Can you work these out from the model? Positions are in its coordinate system, mm. Face numbers are marked on the shaded views. A direction names the side the tool comes from. Round coordinates to 2 decimals unless told otherwise and drop trailing zeros. Loops run counter-clockwise (first coordinate to the right, second up) from the corner with the lowest first, then second, coordinate; pieces in that order, holes last.
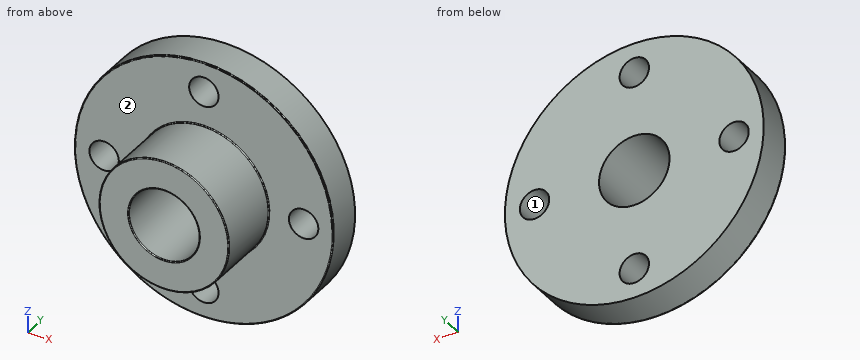
from build123d import *

# Parameters (mm, degrees)
F2_R     = 19.05
F3_DEPTH = 63.5
F4_R     = 7.9375
F5_DEPTH = 127
F6_DEPTH = 25.4
F7_R     = 0.508
F8_R     = 0.508


with BuildPart() as f1:
    # F0 (on Right) → F1 (revolve)
    with BuildSketch(Plane.YZ):
        Polygon((0, 35.052), (0, 0), (53.848, 0), (53.848, 69.85), (34.798, 69.85), (34.798, 35.052), align=None)
    revolve(axis=Axis((0, 26.924, 0), (0, -1, 0)))

    # F2 (on face) → F3 (cut, symmetric)
    with BuildSketch(Plane.XZ.offset(-34.798)):
        Circle(F2_R)
    extrude(amount=F3_DEPTH, both=True, mode=Mode.SUBTRACT)

    # F4 (on face) → F5 (cut)
    with BuildSketch(Plane.XZ.offset(-34.798)):
        with Locations((0, 53.848)):
            Circle(F4_R)
        with Locations((-53.848, 0)):
            Circle(F4_R)
        with Locations((0, -53.848)):
            Circle(F4_R)
        with Locations((53.848, 0)):
            Circle(F4_R)
    extrude(amount=-F5_DEPTH, mode=Mode.SUBTRACT)

    # F4 (on face) → F6 (cut)
    with BuildSketch(Plane.XZ.offset(-34.798)):
        with Locations((0, 53.848)):
            Circle(F4_R)
        with Locations((-53.848, 0)):
            Circle(F4_R)
        with Locations((0, -53.848)):
            Circle(F4_R)
        with Locations((53.848, 0)):
            Circle(F4_R)
    extrude(amount=-F6_DEPTH, mode=Mode.SUBTRACT)

    # F7
    f7_edges = [f1.edges().sort_by_distance(p)[0] for p in [
        (-19.05, 0, 0),
    ]]
    fillet(f7_edges, radius=F7_R)

    # F8
    f8_edges = [f1.edges().sort_by_distance(p)[0] for p in [
        (0, 0, -35.052),
        (0, 34.798, -35.052),
        (0, 34.798, -69.85),
    ]]
    fillet(f8_edges, radius=F8_R)


solid = f1.part
(1) For the marked faces 1 and 2, which set-ups out of +Z, -Z, +X, -X, +Y, -Y let a thin tool reach every point of the face, with its end or its side?
Worked answers:
face 1: +Y, -Y
face 2: -Y
(2) If we section it at D-D, the plane y = 43: State how many separate pieces and enclosed holes the cut face has, then the cut area to 3 significant figures.
Worked answers:
separate pieces: 1
enclosed holes: 5
area: 13,400 mm2
(3) If I drill on line 1 (Z direction, x = 0, y = 46.5); line 2 (Z direction, x = 0, y = 21); line 3 (Y direction, x = 31, z = 16.5), over which ranges is the centre line in solid material (lowest first)?
Worked answers:
line 1: z = -69.85 to -61.79, -45.91 to -19.05, 19.05 to 45.91, 61.79 to 69.85
line 2: z = -35.05 to -19.05, 19.05 to 35.05
line 3: y = 34.54 to 53.85
(4) If we section it at C-C, the plane y = 15.5: List the corners of the cut face in (x, z) for me.
Worked answers:
outline: circle Ø70.1 at (0, 0); hole circle Ø38.1 at (0, 0)
(5) If we section it at B-B, the plane z = 0: List the corners of the cut face in (x, y) for me.
Worked answers:
outline: (-69.85, 35.31) arc R0.51 ccw to (-69.34, 34.8) - (-61.79, 34.8) - (-61.79, 53.85) - (-69.85, 53.85) - close; (-45.91, 34.8) - (-35.56, 34.8) arc R0.51 cw to (-35.05, 34.29) - (-35.05, 0.51) arc R0.51 ccw to (-34.54, 0) - (-19.56, 0) arc R0.51 ccw to (-19.05, 0.51) - (-19.05, 53.85) - (-45.91, 53.85) - close; (19.05, 0.51) arc R0.51 ccw to (19.56, 0) - (34.54, 0) arc R0.51 ccw to (35.05, 0.51) - (35.05, 34.29) arc R0.51 cw to (35.56, 34.8) - (45.91, 34.8) - (45.91, 53.85) - (19.05, 53.85) - close; (61.79, 34.8) - (69.34, 34.8) arc R0.51 ccw to (69.85, 35.31) - (69.85, 53.85) - (61.79, 53.85) - close
(6) Will these pins go through, and if not, where does the flat tip stop? P1, Ø2, axis at x = 4, y = 21, coming from the +Z side; P2, Ø2, axis at x = 6, y = 7.5, coming from the +Z side; P3, Ø5, axis at y = 32, z = -53.5, coming from the -X side; P4, Ø18.5, axis at x = 0, z = 53.848, coming from the -Y side.
Worked answers:
P1: stops at z = 34.92
P2: stops at z = 34.69
P3: passes through
P4: stops at y = 34.8
(7) If we section it at A-A, the plane x = 0: List the corners of the cut face in (y, z) for me.
Worked answers:
outline: (0, -34.54) arc R0.51 ccw to (0.51, -35.05) - (34.29, -35.05) arc R0.51 cw to (34.8, -35.56) - (34.8, -45.91) - (53.85, -45.91) - (53.85, -19.05) - (0.51, -19.05) arc R0.51 ccw to (0, -19.56) - close; (0, 19.56) arc R0.51 ccw to (0.51, 19.05) - (53.85, 19.05) - (53.85, 45.91) - (34.8, 45.91) - (34.8, 35.56) arc R0.51 cw to (34.29, 35.05) - (0.51, 35.05) arc R0.51 ccw to (0, 34.54) - close; (34.8, -69.34) arc R0.51 ccw to (35.31, -69.85) - (53.85, -69.85) - (53.85, -61.79) - (34.8, -61.79) - close; (34.8, 61.79) - (53.85, 61.79) - (53.85, 69.85) - (35.31, 69.85) arc R0.51 ccw to (34.8, 69.34) - close
